Check sheet for the modelled part. Datum: model origin and axes. Units: mm. A direction names the side the tool comes from. Give positions to 0.01 mm unless a question says otherwise; leave off trailing zeros. Order: outer loops, then holes, each group sorted by start corner. A loop starts at its lowest first (then second) coordinate and runs counter-clockwise, first axis right, second up. Notation, with made-up numbers: (-28, 21.25) -> (17, 21.25) arc R16 cw to (17, 40.25) -> close; hole circle Ø2 at (62.25, 5). An arc over 180 degrees is marked (long way). Write each question's results on one line, items separated by ' | '.
from build123d import *

# Parameters (mm, degrees)
SKETCH1_R           = 125
BOSS_EXTRUDE1_DEPTH = 5
CUT_EXTRUDE1_REACH  = 7
SKETCH2_R           = 2
CUT_EXTRUDE2_REACH  = 7
CUT_EXTRUDE3_REACH  = 7
SKETCH4_W           = 10
SKETCH4_H           = 80
CUT_EXTRUDE4_REACH  = 7


with BuildPart() as part:
    # Sketch1 → Boss-Extrude1 (new body)
    with BuildSketch(Plane.XY):
        Circle(SKETCH1_R)
    extrude(amount=BOSS_EXTRUDE1_DEPTH)

    # Sketch2 → Cut-Extrude1 (cut, up to next)
    with BuildSketch(Plane.XY.offset(5), mode=Mode.PRIVATE) as cut_extrude1_sk1:
        with Locations((-56.464466094, -63.535533906)):
            Circle(SKETCH2_R)
    cut_extrude1_tool1 = extrude(cut_extrude1_sk1.sketch, amount=-CUT_EXTRUDE1_REACH, mode=Mode.PRIVATE) & part.part
    add(cut_extrude1_tool1.solids().sort_by_distance((-56.464466, -63.535534, 5))[0], mode=Mode.SUBTRACT)
    # Sketch2 → Cut-Extrude1 (cut, up to next)
    with BuildSketch(Plane.XY.offset(5), mode=Mode.PRIVATE) as cut_extrude1_sk2:
        with Locations((-63.535533906, -56.464466094)):
            Circle(SKETCH2_R)
    cut_extrude1_tool2 = extrude(cut_extrude1_sk2.sketch, amount=-CUT_EXTRUDE1_REACH, mode=Mode.PRIVATE) & part.part
    add(cut_extrude1_tool2.solids().sort_by_distance((-63.535534, -56.464466, 5))[0], mode=Mode.SUBTRACT)
    # Sketch2 → Cut-Extrude1 (cut, up to next)
    with BuildSketch(Plane.XY.offset(5), mode=Mode.PRIVATE) as cut_extrude1_sk3:
        with Locations((-56.464466094, 63.535533906)):
            Circle(SKETCH2_R)
    cut_extrude1_tool3 = extrude(cut_extrude1_sk3.sketch, amount=-CUT_EXTRUDE1_REACH, mode=Mode.PRIVATE) & part.part
    add(cut_extrude1_tool3.solids().sort_by_distance((-56.464466, 63.535534, 5))[0], mode=Mode.SUBTRACT)
    # Sketch2 → Cut-Extrude1 (cut, up to next)
    with BuildSketch(Plane.XY.offset(5), mode=Mode.PRIVATE) as cut_extrude1_sk4:
        with Locations((-63.535533906, 56.464466094)):
            Circle(SKETCH2_R)
    cut_extrude1_tool4 = extrude(cut_extrude1_sk4.sketch, amount=-CUT_EXTRUDE1_REACH, mode=Mode.PRIVATE) & part.part
    add(cut_extrude1_tool4.solids().sort_by_distance((-63.535534, 56.464466, 5))[0], mode=Mode.SUBTRACT)
    # Sketch2 → Cut-Extrude1 (cut, up to next)
    with BuildSketch(Plane.XY.offset(5), mode=Mode.PRIVATE) as cut_extrude1_sk5:
        with Locations((56.464466094, 63.535533906)):
            Circle(SKETCH2_R)
    cut_extrude1_tool5 = extrude(cut_extrude1_sk5.sketch, amount=-CUT_EXTRUDE1_REACH, mode=Mode.PRIVATE) & part.part
    add(cut_extrude1_tool5.solids().sort_by_distance((56.464466, 63.535534, 5))[0], mode=Mode.SUBTRACT)
    # Sketch2 → Cut-Extrude1 (cut, up to next)
    with BuildSketch(Plane.XY.offset(5), mode=Mode.PRIVATE) as cut_extrude1_sk6:
        with Locations((63.535533906, 56.464466094)):
            Circle(SKETCH2_R)
    cut_extrude1_tool6 = extrude(cut_extrude1_sk6.sketch, amount=-CUT_EXTRUDE1_REACH, mode=Mode.PRIVATE) & part.part
    add(cut_extrude1_tool6.solids().sort_by_distance((63.535534, 56.464466, 5))[0], mode=Mode.SUBTRACT)
    # Sketch2 → Cut-Extrude1 (cut, up to next)
    with BuildSketch(Plane.XY.offset(5), mode=Mode.PRIVATE) as cut_extrude1_sk7:
        with Locations((63.535533906, -56.464466094)):
            Circle(SKETCH2_R)
    cut_extrude1_tool7 = extrude(cut_extrude1_sk7.sketch, amount=-CUT_EXTRUDE1_REACH, mode=Mode.PRIVATE) & part.part
    add(cut_extrude1_tool7.solids().sort_by_distance((63.535534, -56.464466, 5))[0], mode=Mode.SUBTRACT)
    # Sketch2 → Cut-Extrude1 (cut, up to next)
    with BuildSketch(Plane.XY.offset(5), mode=Mode.PRIVATE) as cut_extrude1_sk8:
        with Locations((56.464466094, -63.535533906)):
            Circle(SKETCH2_R)
    cut_extrude1_tool8 = extrude(cut_extrude1_sk8.sketch, amount=-CUT_EXTRUDE1_REACH, mode=Mode.PRIVATE) & part.part
    add(cut_extrude1_tool8.solids().sort_by_distance((56.464466, -63.535534, 5))[0], mode=Mode.SUBTRACT)

    # Sketch3 → Cut-Extrude2 (cut, up to next)
    with BuildSketch(Plane.XY.offset(5), mode=Mode.PRIVATE) as cut_extrude2_sk1:
        with BuildLine():
            Line((-91.651513899, -85), (91.651513899, -85))
            ThreePointArc((91.651513899, -85), (0, -125), (-91.651513899, -85))
        make_face()
    cut_extrude2_tool1 = extrude(cut_extrude2_sk1.sketch, amount=-CUT_EXTRUDE2_REACH, mode=Mode.PRIVATE) & part.part
    add(cut_extrude2_tool1.solids().sort_by_distance((0, -101.241971, 5))[0], mode=Mode.SUBTRACT)

    # Sketch4 → Cut-Extrude3 (cut, up to next)
    with BuildSketch(Plane.XY.offset(5), mode=Mode.PRIVATE) as cut_extrude3_sk1:
        with Locations((93, -14)):
            Rectangle(SKETCH4_W, SKETCH4_H)
    cut_extrude3_tool1 = extrude(cut_extrude3_sk1.sketch, amount=-CUT_EXTRUDE3_REACH, mode=Mode.PRIVATE) & part.part
    add(cut_extrude3_tool1.solids().sort_by_distance((93, -14, 5))[0], mode=Mode.SUBTRACT)

    # Sketch5 → Cut-Extrude4 (cut, up to next)
    with BuildSketch(Plane.XY.offset(5), mode=Mode.PRIVATE) as cut_extrude4_sk1:
        with BuildLine():
            ThreePointArc((75, 100), (0, 125), (-75, 100))
            Line((-75, 100), (75, 100))
        make_face()
    cut_extrude4_tool1 = extrude(cut_extrude4_sk1.sketch, amount=-CUT_EXTRUDE4_REACH, mode=Mode.PRIVATE) & part.part
    add(cut_extrude4_tool1.solids().sort_by_distance((0, 110.090997, 5))[0], mode=Mode.SUBTRACT)


solid = part.part
1. Material ranges on probe 1 along X at (y, z) = (-2, 0.6); probe 2 along X at (y, z) = (-29, 1.05); probe 3 along Y at (x, z) = (83, 2.95), recorded low to high. Write a range as from..to.
Verdict:
probe 1: x = -124.98..88, 98..124.98 | probe 2: x = -121.59..88, 98..121.59 | probe 3: y = -85..93.47
2. Section check C-C on y = -47. Record the cut outline in (x, z), then the cut area to 3 significant figures.
Verdict:
outline: (-115.83, 0) -> (88, 0) -> (88, 5) -> (-115.83, 5) -> close; (98, 0) -> (115.83, 0) -> (115.83, 5) -> (98, 5) -> close | area: 1,110 mm^2
3. Access from +Z, -Z, +X, -X, +Y, -Y to the whole of each face (thin tool, end or side, straight path). Record for faces 1 (the flat face through (98, -15, 3)), 2 (the cylindrical face through (124.62, 9.75, 2.46)).
Verdict:
face 1: +Z, -Z | face 2: +Z, -Z, +X
4. Section check A-A on y = -13. Record the cut outline in (x, z).
Verdict:
outline: (-124.32, 0) -> (88, 0) -> (88, 5) -> (-124.32, 5) -> close; (98, 0) -> (124.32, 0) -> (124.32, 5) -> (98, 5) -> close
5. Mould release check, pull along Y, two halves, no side actions. Record for faces 3 (the flat face through (93, -54, 3)), 4 (the flat face through (-2, 9, 5)), 5 (the cylindrical face through (-124.357, 12.665, 2.465)): +Y half, -Y half, draft (parallel to the pull), parting line (faces both ways), or undercut.
Verdict:
face 3: undercut | face 4: draft | face 5: parting line
6. Gauge pin test, flat ends, axial feed: pin 1 Ø5 at (x, y) = (56.46, -63.54) entering from -Z; pin 2 Ø3 at (y, z) = (-35, 2) entering from -X; pin 3 Ø1.5 at (x, z) = (93, 1.5) entering from -Y; pin 4 Ø2.5 at (x, y) = (-63.54, 56.46) entering from -Z. Record the tip position at first contact, or that the pin passes through.
Verdict:
pin 1: stops at z = 0 | pin 2: stops at x = -120.43 | pin 3: stops at y = -84.35 | pin 4: passes through
7. Section check D-D on x = -79.5. Record the cut outline in (y, z), then the cut area to 3 significant figures.
Verdict:
outline: (-85, 0) -> (96.46, 0) -> (96.46, 5) -> (-85, 5) -> close | area: 907 mm^2
8. Section check B-B on z = 1. Give the number of separate pieces and of enclosed holes in the cut face, then the cut area to 3 significant figures.
Verdict:
separate pieces: 1 | enclosed holes: 9 | area: 40,600 mm^2
